```python
from build123d import *

# Parameters (mm, degrees)
F0_W     = 50
F0_H     = 50
F1_DEPTH = 17
F2_T     = -2.5
F3_R     = 21
F4_DEPTH = 1


with BuildPart() as f1:
    # F0 (on Top) → F1 (new body)
    with BuildSketch(Plane.XY):
        Rectangle(F0_W, F0_H)
    extrude(amount=F1_DEPTH)

    # F2
    f2_openings = [f1.faces().sort_by_distance(p)[0] for p in [
        (0, -25, 8.5),
    ]]
    offset(amount=F2_T, openings=f2_openings)

    # F3 (on face) → F4 (cut)
    with BuildSketch(Plane.XY.offset(2.5)):
        Circle(F3_R)
    extrude(amount=-F4_DEPTH, mode=Mode.SUBTRACT)


solid = f1.part
```
Build history of the part. All positions in model axes, mm. A direction names the side the tool comes from. Round coordinates to 2 decimals unless told otherwise and drop trailing zeros. Loops run counter-clockwise (first coordinate to the right, second up) from the corner with the lowest first, then second, coordinate; pieces in that order, holes last.
Item 1: Which spindle directions (+Z, -Z, +X, -X, +Y, -Y) get a long thin tool onto all of the face, cutting with end or side? Do faces 1 (the face through (0, 0, 17)), 2 (the face through (-22.5, -2, 8)). Say none if no direction does.
Item 2: Pin check, flat tips, straight feed: P1, Ø22.5, axis at x = 3, y = -12.5, coming from the -Z side; P2, Ø1, axis at x = -2.5, z = 11.5, coming from the -Y side. Stop position of each tip, or through.
Item 3: Drill centre lines: line 1 along Z through (x, y) = (-18, -22); line 2 along Y through (x, z) = (0, 2.3); line 3 along X through (y, z) = (-15.5, 8.25). Where is each one in solid material? Low to high.
Item 4: Saw through at A-A (y = 0). List the corners of the cut face in (x, z), then the cut area to 3 significant figures.
Item 5: Saw through at B-B (z = 4). List the corners of the cut face in (x, y).
Item 6: Saw through at C-C (x = 0). List the corners of the cut face in (y, z), then the cut area to 3 significant figures.
Item 7: Two-plate mould, pull along Y, no slides. Class faces 3 (the face through (0, -1, 14.5)), 4 (the face through (20.03, 6.31, 2.01)), 5 (the face through (0, 22.5, 8)), 6 (the face through (0, 0, 1.5)): released by +Y, released by -Y, zero draft, split by the parting line, or undercut.
Item 8: Saw through at D-D (y = 11.5). List the corners of the cut face in (x, z), then the cut area to 3 significant figures.
Worked answers:
1. face 1: +Z, +X, -X, +Y, -Y
1. face 2: -Y
2. P1: stops at z = 0
2. P2: stops at y = 22.5
3. line 1: z = 0 to 2.5, 14.5 to 17
3. line 2: y = -25 to -21, 21 to 25
3. line 3: x = -25 to -22.5, 22.5 to 25
4. outline: (-25, 0) - (25, 0) - (25, 17) - (-25, 17) - close; hole (-22.5, 2.5) - (-21, 2.5) - (-21, 1.5) - (21, 1.5) - (21, 2.5) - (22.5, 2.5) - (22.5, 14.5) - (-22.5, 14.5) - close
4. area: 268 mm2
5. outline: (-25, -25) - (-22.5, -25) - (-22.5, 22.5) - (22.5, 22.5) - (22.5, -25) - (25, -25) - (25, 25) - (-25, 25) - close
6. outline: (-25, 0) - (25, 0) - (25, 17) - (-25, 17) - (-25, 14.5) - (22.5, 14.5) - (22.5, 2.5) - (21, 2.5) - (21, 1.5) - (-21, 1.5) - (-21, 2.5) - (-25, 2.5) - close
6. area: 238 mm2
7. face 3: zero draft
7. face 4: undercut
7. face 5: released by -Y
7. face 6: undercut
8. outline: (-25, 0) - (25, 0) - (25, 17) - (-25, 17) - close; hole (-22.5, 2.5) - (-17.57, 2.5) - (-17.57, 1.5) - (17.57, 1.5) - (17.57, 2.5) - (22.5, 2.5) - (22.5, 14.5) - (-22.5, 14.5) - close
8. area: 275 mm2
